The listing builds one solid part. Answer for the finished solid, in the listing's coordinates (mm). A direction names the side the tool comes from. Round coordinates to 2 decimals unless told otherwise and drop trailing zeros. Write each loop counter-clockwise with the first axis right and the second up, starting at its lowest first coordinate (ties: lowest second). Pieces come first, ordered by that corner, then holes.
(1) Each of these flat-tipped pins is pushed along its axis until it touches: pin 1 Ø1 at (x, y) = (-11.5, 3.5) entering from +Z; pin 2 Ø4.5 at (x, z) = (4, -39.5) entering from +Y; pin 3 Ø1.5 at (x, z) = (7.5, -8.5) entering from +Y. Where does it stop, or does it pass through?
(2) A cutting plane is placed at C-C, the plane y = 6.75. Give the vertices of the cut face in (x, z), and give its area (3 significant figures).
(3) Find the intervals of material crossed by probe 1 along Z at (x, y) = (0.5, 13); probe 2 along X at (y, z) = (7.5, -7.5); probe 3 along Z at (x, y) = (-9, 4.75), in increasing order.
(4) A cutting plane is placed at B-B, the plane z = -37. Give the vertices of the cut face in (x, y).
(5) For faces 4 (the face through (-1, 10, -26.65)), 5 (the face through (0.07, 1.01, 35.35)), 6 (the face through (41, 10, 24.15)), 7 (the face through (0, 2, 34)), determine the directions among +Z, -Z, +X, -X, +Y, -Y from which every point of the face is accessible in a straight line to the end or side of a thin tool.
(6) The mould has two halves that part along Z. Classify faces 1 (the face through (0, 1, -45)), 2 (the face through (-10, 15, -27)), 3 (the face through (-37.15, 4, 0)): +Z half, -Z half, draft (parallel to the pull), parting line (faces both ways), or undercut.
(7) A cutting plane is placed at D-D, the plane z = 10. Give the vertices of the cut face in (x, y).
(8) A cutting plane is placed at A-A, the plane x = 0. Give the vertices of the cut face in (y, z), and give its area (3 significant figures).
from build123d import *

# Parameters (mm, degrees)
CROQUIS2_W              = 85
CROQUIS2_H              = 60
SALIENTE_EXTRUIR1_DEPTH = 15
VACIADO1_T              = -3
CROQUIS3_W              = 79
CROQUIS3_H              = 54
CROQUIS3_W_2            = 78.3
CROQUIS3_H_2            = 53.3
SALIENTE_EXTRUIR2_DEPTH = 12
CROQUIS6_W              = 3.35
CROQUIS6_H              = 48.3
CORTAR_EXTRUIR2_DEPTH   = 12
SALIENTE_EXTRUIR4_DEPTH = 2
SALIENTE_EXTRUIR5_DEPTH = 2
CROQUIS9_R              = 1.65
CORTAR_EXTRUIR3_DEPTH   = 21


with BuildPart() as part:
    # Croquis2 → Saliente-Extruir1 (new body)
    with BuildSketch(Plane(origin=(0, 0, 0), x_dir=(1, 0, 0), z_dir=(0, 1, 0))):
        Rectangle(CROQUIS2_W, CROQUIS2_H)
    extrude(amount=SALIENTE_EXTRUIR1_DEPTH)

    # Vaciado1
    vaciado1_openings = [part.faces().sort_by_distance(p)[0] for p in [
        (0, 15, 0),
    ]]
    offset(amount=VACIADO1_T, openings=vaciado1_openings, kind=Kind.INTERSECTION)

    # Croquis3 → Saliente-Extruir2 (add)
    with BuildSketch(Plane(origin=(0, 3, 0), x_dir=(1, 0, 0), z_dir=(0, 1, 0))):
        Rectangle(CROQUIS3_W, CROQUIS3_H)
        Rectangle(CROQUIS3_W_2, CROQUIS3_H_2, mode=Mode.SUBTRACT)
    extrude(amount=SALIENTE_EXTRUIR2_DEPTH)

    # Croquis6 → Cortar-Extruir2 (cut)
    with BuildSketch(Plane(origin=(0, 15, 0), x_dir=(1, 0, 0), z_dir=(0, 1, 0))):
        with Locations((40.825, 0)):
            Rectangle(CROQUIS6_W, CROQUIS6_H)
    extrude(amount=-CORTAR_EXTRUIR2_DEPTH, mode=Mode.SUBTRACT)

    # Croquis7 → Saliente-Extruir4 (add)
    with BuildSketch(Plane(origin=(0, 3, 0), x_dir=(1, 0, 0), z_dir=(0, 1, 0))):
        Polygon((39.15, -26.65), (39.15, -24.15), (42.5, -24.15), (42.5, 24.15), (39.15, 24.15), (39.15, 26.65), (-39.15, 26.65), (-39.15, -26.65), align=None)
        Polygon((37.15, -24.65), (37.15, -22.15), (40.5, -22.15), (40.5, 22.15), (37.15, 22.15), (37.15, 24.65), (-37.15, 24.65), (-37.15, -24.65), align=None, mode=Mode.SUBTRACT)
    extrude(amount=SALIENTE_EXTRUIR4_DEPTH)

    # Croquis8 → Saliente-Extruir5 (add)
    with BuildSketch(Plane.XZ):
        with BuildLine():
            Line((-15, -30), (-15, 30))
            ThreePointArc((-15, 30), (0, 45), (15, 30))
            Line((15, 30), (15, -30))
            ThreePointArc((15, -30), (0, -45), (-15, -30))
        make_face()
    extrude(amount=-SALIENTE_EXTRUIR5_DEPTH)

    # Croquis9 → Cortar-Extruir3 (cut)
    with BuildSketch(Plane(origin=(0, 2, 0), x_dir=(1, 0, 0), z_dir=(0, 1, 0))):
        with Locations(Location((0, 37, 0), (0, 0, 270))):
            Circle(CROQUIS9_R)
        with Locations(Location((0, -37, 0), (0, 0, 270))):
            Circle(CROQUIS9_R)
    extrude(amount=-CORTAR_EXTRUIR3_DEPTH, mode=Mode.SUBTRACT)


solid = part.part
Solutions:
1. pin 1: stops at z = 30
1. pin 2: stops at y = 2
1. pin 3: stops at y = 3
2. outline: (-42.5, -30) - (42.5, -30) - (42.5, -24.15) - (39.15, -24.15) - (39.15, -26.65) - (-39.15, -26.65) - (-39.15, 26.65) - (39.15, 26.65) - (39.15, 24.15) - (42.5, 24.15) - (42.5, 30) - (-42.5, 30) - close
2. area: 765 mm2
3. probe 1: z = -30 to -26.65, 26.65 to 30
3. probe 2: x = -42.5 to -39.15
3. probe 3: z = -30 to -24.65, 24.65 to 30
4. outline: (-13.27, 0) - (-1.65, 0) - (-1.65, 2) - (-13.27, 2) - close; (1.65, 0) - (13.27, 0) - (13.27, 2) - (1.65, 2) - close
5. face 4: +Y
5. face 5: +Y, -Y
5. face 6: +X, +Y
5. face 7: +Z, +X, -X, +Y
6. face 1: -Z half
6. face 2: draft
6. face 3: undercut
7. outline: (-42.5, 0) - (42.5, 0) - (42.5, 5) - (40.5, 5) - (40.5, 3) - (-37.15, 3) - (-37.15, 5) - (-39.15, 5) - (-39.15, 15) - (-42.5, 15) - close
8. outline: (0, -45) - (2, -45) - (2, -38.65) - (0, -38.65) - close; (0, -35.35) - (2, -35.35) - (2, -30) - (15, -30) - (15, -26.65) - (5, -26.65) - (5, -24.65) - (3, -24.65) - (3, 24.65) - (5, 24.65) - (5, 26.65) - (15, 26.65) - (15, 30) - (2, 30) - (2, 35.35) - (0, 35.35) - close; (0, 38.65) - (2, 38.65) - (2, 45) - (0, 45) - close
8. area: 315 mm2
